The model under review builds one solid part; all positions refer to its coordinate system, in mm. Give positions to 0.01 mm unless a question says otherwise; leave off trailing zeros. Order: outer loops, then holes, each group sorted by start corner. A loop starts at its lowest first (then second) coordinate and runs counter-clockwise, first axis right, second up.
```python
from build123d import *

# Parameters (mm, degrees)
BOSS_EXTRUDE1_DEPTH = 5.8674
SKETCH2_R           = 3.175
CUT_EXTRUDE2_DEPTH  = 10.16
SKETCH4_R           = 3.175
CUT_EXTRUDE3_DEPTH  = 10.16


with BuildPart() as part:
    # Sketch1 → Boss-Extrude1 (new body)
    with BuildSketch(Plane(origin=(0, 0, 0), x_dir=(1, 0, 0), z_dir=(0, 1, 0))):
        Polygon((0, 0), (233.866472168, 0), (233.866472168, 15.870150114), (220.6625, 29.074122282), (0, 29.074122282), (-220.662333268, 29.345384182), (-234.132717449, 15.875), (-234.132717449, 0), align=None)
    extrude(amount=BOSS_EXTRUDE1_DEPTH)

    # Sketch2 → Cut-Extrude2 (cut)
    with BuildSketch(Plane.XZ):
        with Locations(Location((-223.020217449, -11.568269312, 0), (0, 0, 270))):
            Circle(SKETCH2_R)
    extrude(amount=-CUT_EXTRUDE2_DEPTH, mode=Mode.SUBTRACT)

    # Sketch4 → Cut-Extrude3 (cut)
    with BuildSketch(Plane.XZ):
        with Locations(Location((222.690472168, -11.294122282, 0), (0, 0, 270))):
            Circle(SKETCH4_R)
    extrude(amount=-CUT_EXTRUDE3_DEPTH, mode=Mode.SUBTRACT)


solid = part.part
```
Item 1: Clearance check with a flat-ended pin moving along its axis: pin 1 Ø3 at (x, y) = (-173, 3.5) entering from -Z. State where the tip first meets the part, or that it passes through.
Values found:
pin 1: stops at z = -29.29
Item 2: For line 1 (X direction, y = 4.55, z = -12); line 2 (X direction, y = 0.7, z = -10); line 3 (Z direction, x = -200, y = 1.65), list the stretches that pass through material, from the lowest coordinate up.
Values found:
line 1: x = -234.13 to -226.17, -219.87 to 219.59, 225.79 to 233.87
line 2: x = -234.13 to -225.78, -220.26 to 219.79, 225.59 to 233.87
line 3: z = -29.32 to 0
Item 3: Take a section at A-A (y = 1.6). Give the number of separate pieces and of enclosed holes in the cut face, and give its area (3 significant figures).
Values found:
separate pieces: 1
enclosed holes: 2
area: 13,400 mm2
Item 4: Take a section at B-B (z = -22). Give the boundary of the cut face in (x, y), and give its area (3 significant figures).
Values found:
outline: (-228.01, 0) - (227.74, 0) - (227.74, 5.87) - (-228.01, 5.87) - close
area: 2,670 mm2
